Check sheet for the drawn part. Datum: minimum x, y, z corner. Units: mm. Round coordinates to 2 decimals unless told otherwise and drop trailing zeros. Write each loop counter-clockwise with the first axis right and the second up, starting at its lowest first coordinate (ties: lowest second). Pieces come first, ordered by that corner, then holes. Notation, with made-up numbers: (25, -4) - (83, -4) arc R6 ccw to (83, 6) - close; hole circle Ø7 at (-17, 88). An arc over 180 degrees is marked (long way). Write each question's results on one line, items separated by ' | '.
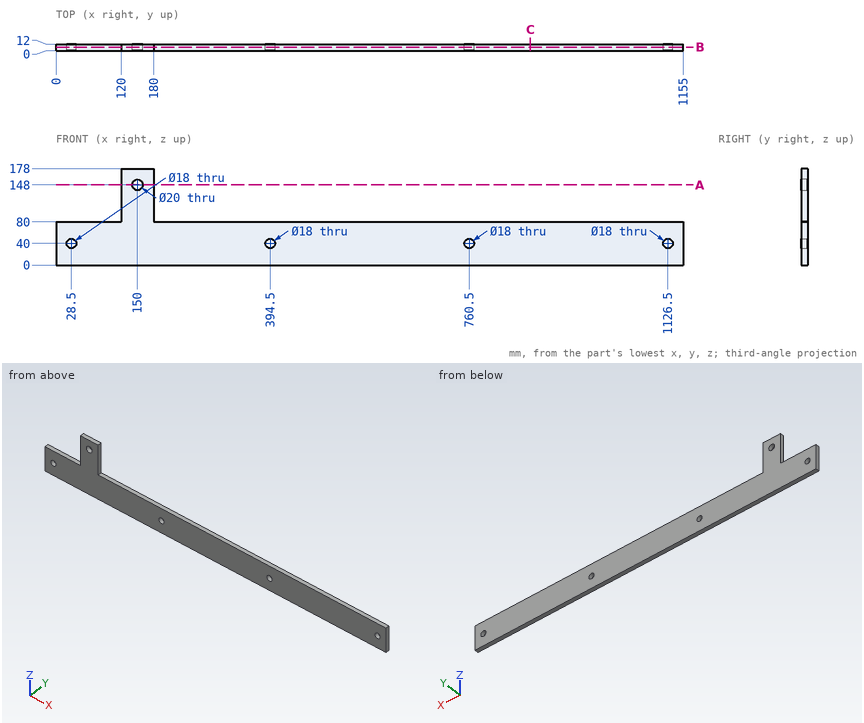
(1) Section check C-C (x = 873). Record the cut outline in (y, z), plus the area to 3 significant figures.
Answer:
outline: (0, 0) - (12, 0) - (12, 80) - (0, 80) - close | area: 960 mm2
(2) Section check A-A (z = 148). Record the cut outline in (x, y), plus the area to 3 significant figures.
Answer:
outline: (120, 0) - (140, 0) - (140, 12) - (120, 12) - close; (160, 0) - (180, 0) - (180, 12) - (160, 12) - close | area: 480 mm2
(3) Section check B-B (y = 6.25). Record the cut outline in (x, z), plus the area to 3 significant figures.
Answer:
outline: (0, 0) - (1155, 0) - (1155, 80) - (180, 80) - (180, 178) - (120, 178) - (120, 80) - (0, 80) - close; hole circle Ø18 at (28.5, 40); hole circle Ø20 at (150, 148); hole circle Ø18 at (394.5, 40); hole circle Ø18 at (760.5, 40); hole circle Ø18 at (1126.5, 40) | area: 96,900 mm2
(4) Go/stop test with flat-tipped pins: pin 1 Ø6 at (y, z) = (8, 118.5) entering from +X; pin 2 Ø10 at (x, z) = (940.5, 58) entering from -Y; pin 3 Ø3 at (y, z) = (4.5, 125) entering from -X. Record where each tip stops, or that it passes through.
Answer:
pin 1: x = 180 | pin 2: y = 0 | pin 3: x = 120
(5) Thickness scan on L1, parallel to X at y = 3.5, z = 40; L2, parallel to Z at x = 150, y = 4; L3, parallel to Z at x = 1126.5, y = 8.75. Record the ranges inside material, lowest first.
Answer:
L1: 0 to 19.5, 37.5 to 385.5, 403.5 to 751.5, 769.5 to 1117.5, 1135.5 to 1155 | L2: 0 to 138, 158 to 178 | L3: 0 to 31, 49 to 80
